from build123d import *

# Parameters (mm, degrees)
BOSS_EXTRUDE1_DEPTH = 2.54
FILLET1_R           = 1.27
CUT_EXTRUDE2_DEPTH  = 2.54


with BuildPart() as part:
    # Sketch1 → Boss-Extrude1 (new body)
    with BuildSketch(Plane(origin=(0, 0, 0), x_dir=(1, 0, 0), z_dir=(0, 1, 0))):
        Polygon((12.7, 0), (0, 0), (-10.16, 0), (-10.16, 5.08), (12.7, 5.08), align=None)
    extrude(amount=BOSS_EXTRUDE1_DEPTH)

    # Fillet1
    fillet1_edges = [part.edges().sort_by_distance(p)[0] for p in [
        (-10.16, 0, -2.54),
        (-10.16, 2.54, -2.54),
    ]]
    fillet(fillet1_edges, radius=FILLET1_R - 0.0001)  # a hair under: the kernel refuses the full size

    # Sketch3 → Cut-Extrude2 (cut)
    with BuildSketch(Plane(origin=(0, 2.54, 0), x_dir=(1, 0, 0), z_dir=(0, 1, 0))):
        Polygon((12.7, 5.08), (10.16, 2.54), (12.7, 0), align=None)
    extrude(amount=-CUT_EXTRUDE2_DEPTH, mode=Mode.SUBTRACT)


solid = part.part
Can you work these out from the model? Positions are in its coordinate system, mm. A direction names the side the tool comes from. Give positions to 0.01 mm unless a question says otherwise; leave off trailing zeros. Loops run counter-clockwise (first coordinate to the right, second up) from the corner with the lowest first, then second, coordinate; pieces in that order, holes last. Notation, with made-up numbers: (88, 45) - (110, 45) arc R17 cw to (110, 73) - close; hole circle Ø10 at (26.25, 55). An arc over 180 degrees is marked (long way). One line per item, written item: value.
(1) If we section it at D-D, the plane y = 1.95: List the corners of the cut face in (x, z) for me, plus the area to 3 significant figures.
Verdict:
outline: (-9.96, -5.08) - (12.7, -5.08) - (10.16, -2.54) - (12.7, 0) - (-9.96, 0) - close
area: 109 mm^2
(2) If we section it at B-B, the plane y = 0.65: List the corners of the cut face in (x, z) for me.
Verdict:
outline: (-10, -5.08) - (12.7, -5.08) - (10.16, -2.54) - (12.7, 0) - (-10, 0) - close
(3) If we mould it in two halves opening along Z, with no side actions, what happens to faces 1 (the face through (11.4, 1.3, -1.3)), 2 (the face through (2, 0, -3)), 3 (the face through (1, 1, 0))? For each: released by +Z, released by -Z, zero draft, split by the parting line, or undercut.
Verdict:
face 1: undercut
face 2: zero draft
face 3: released by +Z
(4) I need wall thicknesses on line 1 along Z through (x, y) = (11.75, 1.35); line 2 along Z through (x, y) = (11.25, 2.3); line 3 along Y through (x, z) = (-9, -3.1). Which ranges of each line are inside material? Lowest first, please.
Verdict:
line 1: -5.08 to -4.13, -0.95 to 0
line 2: -5.08 to -3.63, -1.45 to 0
line 3: 0 to 2.54
(5) On a 3-axis mill with a long thin cutter (end or side, diameter ignored), from which of +Z, -Z, +X, -X, +Y, -Y can I reach the whole of each face in a straight line? I mean faces 4 (the face through (-9.798, 2.158, -2.576)), 5 (the face through (11.45, 1.29, -3.83)). Say none if no direction works.
Verdict:
face 4: +Z, -Z, -X, +Y
face 5: +X, +Y, -Y
